Design review of the part shown in the three views and the two pictorial views. Dimensions are in mm from the part's minimum x, y and z. A direction names the side the tool comes from. Coordinates: 2 decimals unless noted, no trailing zeros. Write each loop counter-clockwise with the first axis right and the second up, starting at its lowest first coordinate (ties: lowest second). Pieces come first, ordered by that corner, then holes. Notation, with made-up numbers: (-5, 3) -> (5, 3) arc R16 ccw to (5, 9) -> close; hole circle Ø5 at (-2, -20.5). An arc over 180 degrees is marked (long way). Answer in a Markdown table with one row per item. Add a question column.
Item 1: Take a section at C-C, the plane z = 8.7. Write out the cut boundary in (x, y).
Item 2: Clearance check with a flat-ended pin moving along its axis: P1, Ø3.5, axis at x = 8.7, z = 8.7, coming from the +Y side. State where the tip first meets the part, or that it passes through.
Item 3: Draft analysis for pull direction Z (two halves, no side actions). For the marked faces 3, 4, 5 and 6, state which applies: released by +Z, released by -Z, zero draft, split by the parting line, or undercut.
Item 4: Take a section at B-B, the plane x = 8.7. Write out the cut boundary in (y, z).
Item 5: To check wall thickness, follow line 1 (X direction, y = 1.25, z = 8.75); line 2 (Z direction, x = 4.5, y = 4.5). State the ranges of each line that lie inside material, in increasing order.
Item 6: Take a section at A-A, the plane y = 2.5. Write out the cut boundary in (x, z).
Item 7: Take a section at D-D, the plane z = 15. Write out the cut boundary in (x, y).
Item 8: For the marked faces 1 and 2, list the 3-axis set-ups (+Z, -Z, +X, -X, +Y, -Y) from which the entire face can be reached by the end or side of a thin tool; tool diameter is ignored.
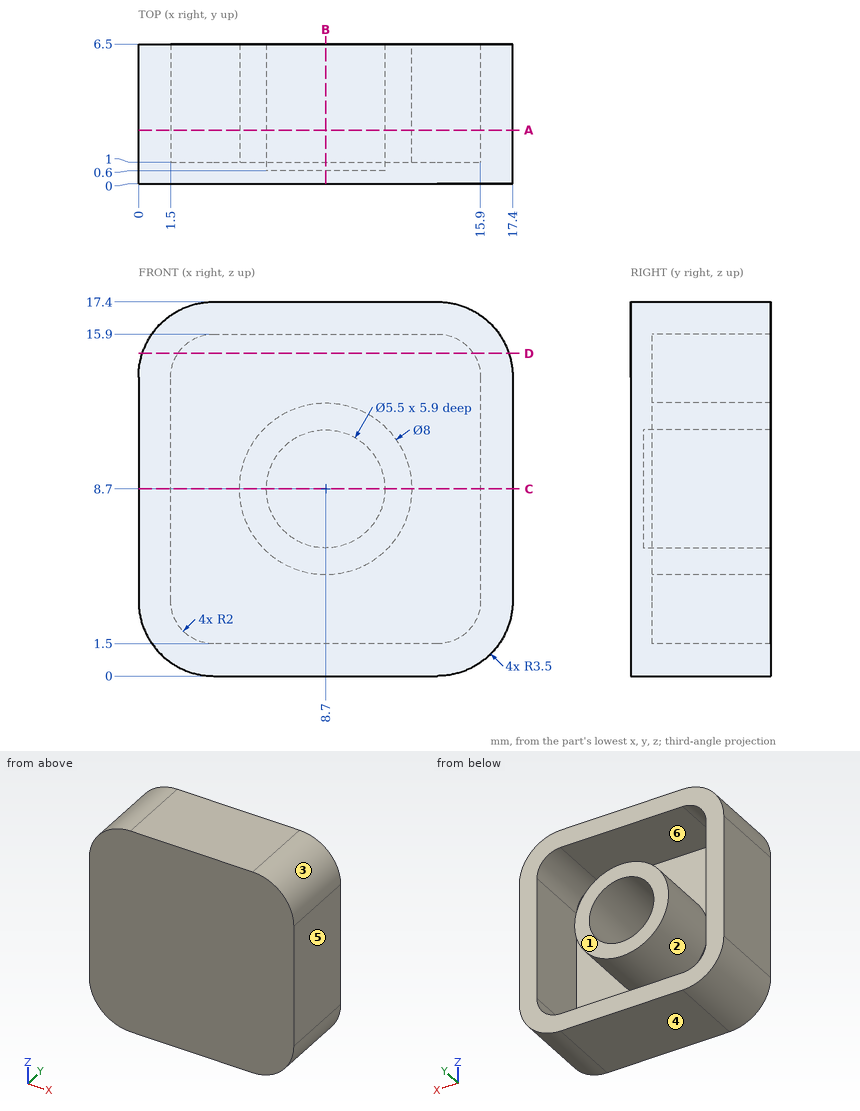
Answers:
| question | item | result |
|---|---|---|
| 1 | outline | (0, 0) -> (17.4, 0) -> (17.4, 6.5) -> (15.9, 6.5) -> (15.9, 1) -> (12.7, 1) -> (12.7, 6.5) -> (11.45, 6.5) -> (11.45, 0.6) -> (5.95, 0.6) -> (5.95, 6.5) -> (4.7, 6.5) -> (4.7, 1) -> (1.5, 1) -> (1.5, 6.5) -> (0, 6.5) -> close |
| 2 | P1 | stops at y = 0.6 |
| 3 | face 3 | released by +Z |
| 3 | face 4 | released by -Z |
| 3 | face 5 | zero draft |
| 3 | face 6 | undercut |
| 4 | outline | (0, 0) -> (6.5, 0) -> (6.5, 1.5) -> (1, 1.5) -> (1, 4.7) -> (6.5, 4.7) -> (6.5, 5.95) -> (0.6, 5.95) -> (0.6, 11.45) -> (6.5, 11.45) -> (6.5, 12.7) -> (1, 12.7) -> (1, 15.9) -> (6.5, 15.9) -> (6.5, 17.4) -> (0, 17.4) -> close |
| 5 | line 1 | x = 0 to 1.5, 4.7 to 5.95, 11.45 to 12.7, 15.9 to 17.4 |
| 5 | line 2 | z = 0 to 1.5, 15.9 to 17.4 |
| 6 | outline | (0, 3.5) arc R3.5 ccw to (3.5, 0) -> (13.9, 0) arc R3.5 ccw to (17.4, 3.5) -> (17.4, 13.9) arc R3.5 ccw to (13.9, 17.4) -> (3.5, 17.4) arc R3.5 ccw to (0, 13.9) -> close; circle Ø8 at (8.7, 8.7); hole (1.5, 3.5) arc R2 ccw to (3.5, 1.5) -> (13.9, 1.5) arc R2 ccw to (15.9, 3.5) -> (15.9, 13.9) arc R2 ccw to (13.9, 15.9) -> (3.5, 15.9) arc R2 ccw to (1.5, 13.9) -> close; hole circle Ø5.5 at (8.7, 8.7) |
| 7 | outline | (0.18, 0) -> (17.22, 0) -> (17.22, 6.5) -> (15.57, 6.5) -> (15.57, 1) -> (1.83, 1) -> (1.83, 6.5) -> (0.18, 6.5) -> close |
| 8 | face 1 | +Z, -Z, +X, -X, +Y |
| 8 | face 2 | +Y |
